Autodesk Inventor part; units mm, degrees
ref_plane "YZ Plane" through (0, 0, 0) normal (1, 0, 0) x (0, 1, 0)
ref_plane "XZ Plane" through (0, 0, 0) normal (0, 1, 0) x (-1, 0, 0)
ref_plane "XY Plane" through (0, 0, 0) normal (0, 0, 1) x (1, 0, 0)
sketch "Sketch1" plane through (0, 0, 0) normal (0, 0, 1) x (1, 0, 0)
  circle A0 centre (-24.0055, -25.7521) radius 3.25
  circle A1 centre (-24.0055, -25.7521) radius 2
  point P0 (0, 0)
  dimension "d0" = 6.5
  dimension "d1" = 4
extrude "Extrusion1" add sketch "Sketch1" along normal blind 1
sketch "Sketch2" plane through (-24.0055, -25.7521, 1) normal (0, 0, 1) x (1, 0, 0)
  circle A0 centre (0, 0) radius 3
  circle A1 centre (0, 0) radius 2
  line L0 (0, 0) -> (-2.75, 0)
  line L1 (-2.75, 0) -> (-2.75, 40)
  line L2 (-2.75, 40) -> (0, 40)
  line L3 (0, 40) -> (0, 0)
  line L4 (0, 0) -> (3, 0)
  line L5 (3, 0) -> (3, 40)
  line L6 (3, 40) -> (0, 40)
  line L7 (0, 40) -> (0, 0)
  point P0 (24.0055, 25.7521)
  point P1 (-2.75, 1.199)
  point P2 (3, 0)
  point P3 (0, 40)
  dimension "d4" = 40
  dimension "d5" = 3
  dimension "d8" = 4
  dimension "d9" = 6
extrude "Extrusion2" add sketch "Sketch2" along normal blind 3 contours L4 A1 L3 A0 | A0 L1 L0 A1 L4 | A0 L3 L6 L5 | L3 A1 L0 L1 A0 | A0 L1 L2 L3
chamfer "Chamfer1" distance 0.245 angle 45 2 edges at (-24.6178, -28.689, 1) (-21.0055, -25.1271, 1)
properties part number "slide_clips_4mm"
Part model, mm, in its own coordinate system. A direction names the side the tool comes from. Round coordinates to 2 decimals unless told otherwise and drop trailing zeros. Order: outer loops, then holes, each group sorted by start corner. A loop starts at its lowest first (then second) coordinate and runs counter-clockwise, first axis right, second up. Notation, with made-up numbers: M 46.5,0.5 L 66.5,0.5 A23 cw 66.5,15.5 Z; hole C 20,-4.5 d5. An arc over 180 degrees is marked long. Put each result on its own line as item: value. Start each with the question number.
1. Drop flat-ended pins along their axis: pin 1 (2 mm diameter, centred on y = -7.5, z = 1, fed in from -X); pin 2 (0.9 mm diameter, centred on y = -11.5, z = 3, fed in from +X); pin 3 (3 mm diameter, centred on x = -24, y = -8, fed in from -Z). Give the stop position or say it passes through.
2. Drill centre lines: probe 1 along Y at (x, z) = (-26.25, 3.2); probe 2 along X at (y, z) = (-16.5, 3.25); probe 3 along Y at (x, z) = (-24.75, 2.6). Where is each one in solid material? Low to high. Write a range as [from, to].
3. Tool access for faces 4 (the face through (-21.003, -24.507, 0.475)), 5 (the face through (-24, -7, 4)): list every direction of +Z, -Z, +X, -X, +Y, -Y with a clear straight run to the whole face (end or side of a thin tool).
4. Slice it at C-C on z = 0.6. List the corners of the cut face in (x, y).
5. Two-plate mould, pull along X, no slides. Class faces 1 (the face through (-22.93, -27.44, 1.97)), 2 (the face through (-21.006, -6, 2)), 3 (the face through (-24.79, -28.776, 1.121)): +X half, -X half, draft (parallel to the pull), parting line (faces both ways), or undercut.
6. Slice it at A-A on z = 3.45. List the corners of the cut face in (x, y).
7. Slice it at B-B on y = 2.5. List the corners of the cut face in (x, z).
Findings:
1. pin 1: x = -26.76
1. pin 2: x = -21.01
1. pin 3: z = 1
2. probe 1: [-27.74, 14.25]
2. probe 2: [-26.76, -21.01]
2. probe 3: [-28.66, -27.61], [-23.9, 14.25]
3. face 4: -Z
3. face 5: +Z, +X, -X, +Y, -Y
4. outline: C -24.01,-25.75 d6.5; hole C -24.01,-25.75 d4
5. face 1: undercut
5. face 2: +X half
5. face 3: parting line
6. outline: M -26.76,-24.55 A3 ccw long -21.01,-25.75 L -21.01,14.25 L -26.76,14.25 Z; hole C -24.01,-25.75 d4
7. outline: M -26.76,1 L -21.01,1 L -21.01,4 L -26.76,4 Z
